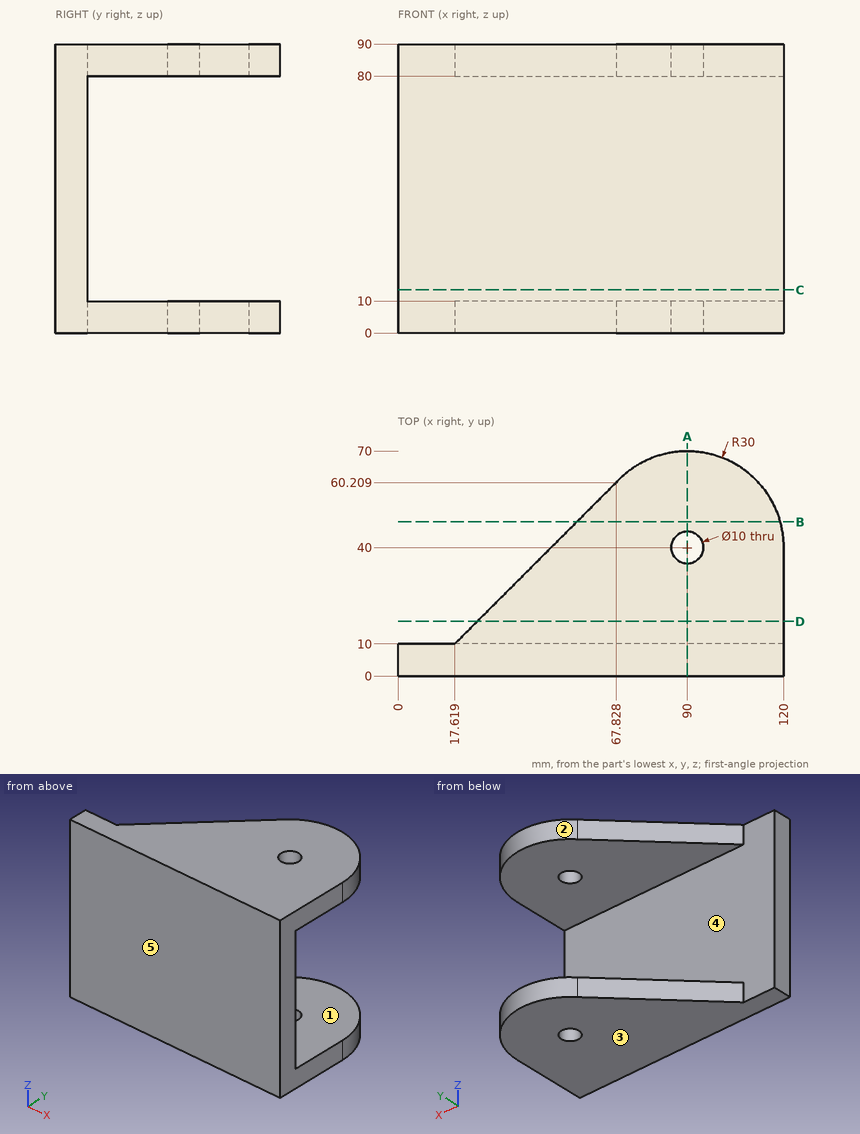
Study the drawing (mm; zero at the part's minimum x, y, z) and answer. A direction names the side the tool comes from. Coordinates: 2 decimals unless noted, no trailing zeros. Order: outer loops, then holes, each group sorted by start corner. A loop starts at its lowest first (then second) coordinate and runs counter-clockwise, first axis right, second up. Notation, with made-up numbers: (63, -20) -> (73, -20) arc R12 cw to (73, -1) -> close; hole circle Ø3 at (18.25, 30.5). An arc over 180 degrees is marked (long way). Answer in a Markdown table with one row per item. Add a question column.
Item 1: Each of these flat-tipped pins is pushed along its axis until it touches: P1, Ø5, axis at x = 93, z = 70, coming from the +Y side; P2, Ø8, axis at x = 90, y = 40, coming from the +Z side. Where does it stop, or does it pass through?
Item 2: Find section B-B (y = 48). Write down the section's boundary in (x, z).
Item 3: Find the intervals of material crossed by L1, parallel to Z at x = 48, y = 24; L2, parallel to Y at x = 90, z = 6.75; L3, parallel to Y at x = 52, z = 30, in increasing order. Write a range as from..to.
Item 4: Find section C-C (z = 13.5). Write down the section's boundary in (x, y).
Item 5: Which of the six approach directions +Z, -Z, +X, -X, +Y, -Y give full straight-line access (tool end or side, diameter ignored) to the marked faces 1 and 2?
Item 6: Determine the mould class of the marked faces 3, 4 and 5 for opening direction Z: +Z half, -Z half, draft (parallel to the pull), parting line (faces both ways), or undercut.
Item 7: Find section A-A (x = 90). Write down the section's boundary in (y, z), then the cut area to 3 significant figures.
Item 8: Find section D-D (y = 17). Write down the section's boundary in (x, z).
Result set:
| question | item | result |
|---|---|---|
| 1 | P1 | stops at y = 10 |
| 1 | P2 | passes through |
| 2 | outline | (55.62, 0) -> (118.91, 0) -> (118.91, 10) -> (55.62, 10) -> close; (55.62, 80) -> (118.91, 80) -> (118.91, 90) -> (55.62, 90) -> close |
| 3 | L1 | z = 0..10, 80..90 |
| 3 | L2 | y = 0..35, 45..70 |
| 3 | L3 | y = 0..10 |
| 4 | outline | (0, 0) -> (120, 0) -> (120, 10) -> (0, 10) -> close |
| 5 | face 1 | +X, -X, +Y |
| 5 | face 2 | +Z, -Z, +Y |
| 6 | face 3 | -Z half |
| 6 | face 4 | undercut |
| 6 | face 5 | draft |
| 7 | outline | (0, 0) -> (35, 0) -> (35, 10) -> (10, 10) -> (10, 80) -> (35, 80) -> (35, 90) -> (0, 90) -> close; (45, 0) -> (70, 0) -> (70, 10) -> (45, 10) -> close; (45, 80) -> (70, 80) -> (70, 90) -> (45, 90) -> close |
| 7 | area | 1,900 mm² |
| 8 | outline | (24.62, 0) -> (120, 0) -> (120, 10) -> (24.62, 10) -> close; (24.62, 80) -> (120, 80) -> (120, 90) -> (24.62, 90) -> close |
